from build123d import *

# Parameters (mm, degrees)
PAD_DEPTH           = 5
PAD001_DEPTH        = 10
POCKET_DEPTH        = 6
SKETCH003_W         = 7
SKETCH003_H         = 4
POCKET001_DEPTH     = 30
SKETCH004_W         = 15
SKETCH004_H         = 5
PAD002_DEPTH        = 10
SKETCH005_W         = 15
SKETCH005_H         = 55
PAD003_DEPTH        = 10
HOLE_D              = 3.4
HOLE_DEPTH          = 25
HOLE_CBORE_D        = 6.1
HOLE_CBORE_DEPTH    = 2.4
HOLE_TIPS_R         = 1.7
SKETCH007_W         = 15
SKETCH007_H         = 5
PAD004_DEPTH        = 10
SKETCH008_W         = 15
SKETCH008_H         = 55
PAD005_DEPTH        = 10
HOLE001_D           = 3.4
HOLE001_DEPTH       = 25
HOLE001_CBORE_D     = 6.1
HOLE001_CBORE_DEPTH = 2.4
HOLE001_TIPS_R      = 1.7
SKETCH010_W         = 15
SKETCH010_H         = 5
PAD006_DEPTH        = 10
SKETCH011_W         = 15
SKETCH011_H         = 55
PAD007_DEPTH        = 10
HOLE002_D           = 3.4
HOLE002_DEPTH       = 25
HOLE002_CBORE_D     = 6.1
HOLE002_CBORE_DEPTH = 2.4
HOLE002_TIPS_R      = 1.7


with BuildPart() as part:
    # Sketch → Pad (new body)
    with BuildSketch(Plane.XY):
        Polygon((77.465972, -44.725), (77.465972, -9.995), (87.465972, -9.995), (87.465972, -50.494492), (0, -100.995), (-87.465972, -50.494492), (-87.465972, 50.494492), (0, 100.995), (96.115509, 100.995), (89.45, 89.45), (0, 89.45), (-77.465972, 44.725), (-77.465972, -44.725), (0, -89.45), align=None)
    extrude(amount=PAD_DEPTH)

    # Sketch001 (on Face16 of Pad) → Pad001 (join)
    with BuildSketch(Plane.XY.offset(5)):
        Polygon((124.090672, 69.449404), (130.75638, 80.99429), (61.475035, 120.995481), (54.809328, 109.450596), align=None)
    extrude(amount=PAD001_DEPTH)

    # Sketch002 (on Face7 of Pad001) → Pocket (cut)
    with BuildSketch(Plane(origin=(0, 0, 5), x_dir=(1, 0, 0), z_dir=(0, 0, -1))):
        Polygon((91.032754, -92.191411), (117.013517, -77.191411), (120.513517, -83.253589), (94.532754, -98.253589), align=None)
    extrude(amount=-POCKET_DEPTH, mode=Mode.SUBTRACT)

    # Sketch003 (on Face8 of Pocket) → Pocket001 (cut)
    with BuildSketch(Plane(origin=(28.354514, -16.370486, 0), x_dir=(0.5, 0.866025, 0), z_dir=(0.866025, -0.5, 0))):
        with Locations((128.856481, 9)):
            Rectangle(SKETCH003_W, SKETCH003_H)
    extrude(amount=-POCKET001_DEPTH, mode=Mode.SUBTRACT)

    # Sketch004 (on Face14 of Pocket001) → Pad002 (join)
    with BuildSketch(Plane.YZ.offset(87.465972)):
        with Locations((-30.244746, 2.5)):
            Rectangle(SKETCH004_W, SKETCH004_H)
    extrude(amount=PAD002_DEPTH)

    # Sketch005 (on Face32 of Pad002) → Pad003 (join)
    with BuildSketch(Plane.YZ.offset(97.465972)):
        with Locations((-30.244746, -22.5)):
            Rectangle(SKETCH005_W, SKETCH005_H)
    extrude(amount=PAD003_DEPTH)

    # Hole
    with Locations(Plane.YZ.offset(107.465972)):
        with Locations((-30.244746, -12.5), (-30.244746, -37.5)):
            CounterBoreHole(HOLE_D / 2, HOLE_CBORE_D / 2, HOLE_CBORE_DEPTH, depth=HOLE_DEPTH)

    # Hole tips → Hole tip 1 section 0
    with BuildSketch(Plane.YZ.offset(82.465972), mode=Mode.PRIVATE) as hole_tip_1_s0:
        with Locations((-30.244746, -12.5)):
            Circle(HOLE_TIPS_R)
    loft([hole_tip_1_s0.sketch, Vertex(81.444509, -30.244746, -12.5)], mode=Mode.SUBTRACT)

    # Hole tips → Hole tip 2 section 0
    with BuildSketch(Plane.YZ.offset(82.465972), mode=Mode.PRIVATE) as hole_tip_2_s0:
        with Locations((-30.244746, -37.5)):
            Circle(HOLE_TIPS_R)
    loft([hole_tip_2_s0.sketch, Vertex(81.444509, -30.244746, -37.5)], mode=Mode.SUBTRACT)

    # Sketch007 (on Face17 of Hole) → Pad004 (join)
    with BuildSketch(Plane(origin=(43.732986, -75.744746, 0), x_dir=(0.866017, 0.500015, 0), z_dir=(0.500015, -0.866017, 0))):
        with Locations((0, 2.5)):
            Rectangle(SKETCH007_W, SKETCH007_H)
    extrude(amount=PAD004_DEPTH)

    # Sketch008 (on Face38 of Pad004) → Pad005 (join)
    with BuildSketch(Plane(origin=(48.733135, -84.404914, 0), x_dir=(0.866017, 0.500015, 0), z_dir=(0.500015, -0.866017, 0))):
        with Locations((0, -22.5)):
            Rectangle(SKETCH008_W, SKETCH008_H)
    extrude(amount=PAD005_DEPTH)

    # Hole001
    with Locations(Plane(origin=(53.733284, -93.065082, 0), x_dir=(0.866017, 0.500015, 0), z_dir=(0.500015, -0.866017, 0))):
        with Locations((0, -12.5), (0, -37.5)):
            CounterBoreHole(HOLE001_D / 2, HOLE001_CBORE_D / 2, HOLE001_CBORE_DEPTH, depth=HOLE001_DEPTH)

    # Hole001 tips → Hole001 tip 1 section 0
    with BuildSketch(Plane(origin=(41.232912, -71.414662, 0), x_dir=(0.866017, 0.500015, 0), z_dir=(0.500015, -0.866017, 0)), mode=Mode.PRIVATE) as hole001_tip_1_s0:
        with Locations((0, -12.5)):
            Circle(HOLE001_TIPS_R)
    loft([hole001_tip_1_s0.sketch, Vertex(40.722165, -70.530058, -12.5)], mode=Mode.SUBTRACT)

    # Hole001 tips → Hole001 tip 2 section 0
    with BuildSketch(Plane(origin=(41.232912, -71.414662, 0), x_dir=(0.866017, 0.500015, 0), z_dir=(0.500015, -0.866017, 0)), mode=Mode.PRIVATE) as hole001_tip_2_s0:
        with Locations((0, -37.5)):
            Circle(HOLE001_TIPS_R)
    loft([hole001_tip_2_s0.sketch, Vertex(40.722165, -70.530058, -37.5)], mode=Mode.SUBTRACT)

    # Sketch010 (on Face20 of Hole001) → Pad006 (join)
    with BuildSketch(Plane(origin=(-43.732986, -75.744746, 0), x_dir=(0.866017, -0.500015, 0), z_dir=(-0.500015, -0.866017, 0))):
        with Locations((0, 2.5)):
            Rectangle(SKETCH010_W, SKETCH010_H)
    extrude(amount=PAD006_DEPTH)

    # Sketch011 (on Face44 of Pad006) → Pad007 (join)
    with BuildSketch(Plane(origin=(-48.733135, -84.404914, 0), x_dir=(0.866017, -0.500015, 0), z_dir=(-0.500015, -0.866017, 0))):
        with Locations((0, -22.5)):
            Rectangle(SKETCH011_W, SKETCH011_H)
    extrude(amount=PAD007_DEPTH)

    # Hole002
    with Locations(Plane(origin=(-53.733284, -93.065082, 0), x_dir=(0.866017, -0.500015, 0), z_dir=(-0.500015, -0.866017, 0))):
        with Locations((0, -36.25), (0, -8.75)):
            CounterBoreHole(HOLE002_D / 2, HOLE002_CBORE_D / 2, HOLE002_CBORE_DEPTH, depth=HOLE002_DEPTH)

    # Hole002 tips → Hole002 tip 1 section 0
    with BuildSketch(Plane(origin=(-41.232912, -71.414662, 0), x_dir=(0.866017, -0.500015, 0), z_dir=(-0.500015, -0.866017, 0)), mode=Mode.PRIVATE) as hole002_tip_1_s0:
        with Locations((0, -36.25)):
            Circle(HOLE002_TIPS_R)
    loft([hole002_tip_1_s0.sketch, Vertex(-40.722165, -70.530058, -36.25)], mode=Mode.SUBTRACT)

    # Hole002 tips → Hole002 tip 2 section 0
    with BuildSketch(Plane(origin=(-41.232912, -71.414662, 0), x_dir=(0.866017, -0.500015, 0), z_dir=(-0.500015, -0.866017, 0)), mode=Mode.PRIVATE) as hole002_tip_2_s0:
        with Locations((0, -8.75)):
            Circle(HOLE002_TIPS_R)
    loft([hole002_tip_2_s0.sketch, Vertex(-40.722165, -70.530058, -8.75)], mode=Mode.SUBTRACT)


solid = part.part
The model under review builds one solid part; all positions refer to its coordinate system, in mm. A direction names the side the tool comes from. Give positions to 0.01 mm unless a question says otherwise; leave off trailing zeros. Loops run counter-clockwise (first coordinate to the right, second up) from the corner with the lowest first, then second, coordinate; pieces in that order, holes last. Notation, with made-up numbers: (51, 58.25) -> (80, 58.25) arc R18 ccw to (80, 83.25) -> close; hole circle Ø6 at (-31, -39.5). An arc over 180 degrees is marked (long way). Answer as a JSON object with one key per item and string values. Group by question number.
Q1. Take a section at C-C (y = 10). Write out the cut boundary in (x, z), plus the area to 3 significant figures.
Q2. Tool access review of faces 1 (the flat face through (-77.466, 1, 2)), 2 (the cylindrical face through (106.283, -27.336, -11.584)), 3 (the flat face through (80, 103, 7)): name each direction out of +Z, -Z, +X, -X, +Y, -Y from which nothing blocks a thin tool from reaching the whole face with its end or side.
Q3. Take a section at B-B (x = -30.5). Write out the cut boundary in (y, z), plus the area to 3 significant figures.
Q4. Insertion check: pin 1 (8 mm diameter, centred on x = 69, z = 6, fed in from -Y); pin 2 (1 mm diameter, centred on x = -57.5, z = -29.5, fed in from +Y); pin 3 (10 mm diameter, centred on x = 70.5, y = 114, fed in from -Z). Each pin has a flat end and moves straight along its axis. Give the tip position at first contact, or say it passes through.
Q5. Take a section at A-A (z = -23.5). Write out the cut boundary in (x, y).
Q6. Wall thickness on line 1 along X through (y, z) = (-89, -9); line 2 along Z through (x, y) = (7, 89.5); line 3 along Z through (x, y) = (102, 88): over which ranges is each line inside the solid? List them lowest first.
Q7. Draft analysis for pull direction Z (two halves, no side actions). For faces 4 (the flat face through (-48.824, -84.352, -24.65)), 5 (the flat face through (40, -67, 0)), 6 (the cylindrical face through (51.775, -86.975, -38.534)), state which applies: pulls with the +Z half, pulls with the -Z half, needs draft (parallel to the pull), parting line crosses it, or undercut.
Answer below:
{
 "1": {"outline": "(-87.47, 0) -> (-77.47, 0) -> (-77.47, 5) -> (-87.47, 5) -> close", "area": "50.0 mm2"},
 "2": {"face 1": "+Z, -Z", "face 2": "+X", "face 3": "none"},
 "3": {"outline": "(-83.39, 0) -> (-71.84, 0) -> (-71.84, 5) -> (-83.39, 5) -> close; (71.84, 0) -> (83.39, 0) -> (83.39, 5) -> (71.84, 5) -> close", "area": "115 mm2"},
 "4": {"pin 1": "stops at y = -63.39", "pin 2": "stops at y = -83.72", "pin 3": "stops at z = 5"},
 "5": {"outline": "(-60.23, -89.31) -> (-47.24, -96.82) -> (-42.24, -88.16) -> (-55.23, -80.65) -> close; (42.24, -88.16) -> (47.24, -96.82) -> (60.23, -89.31) -> (55.23, -80.65) -> close; (97.47, -37.74) -> (107.47, -37.74) -> (107.47, -22.74) -> (97.47, -22.74) -> close"},
 "6": {"line 1": "x = -60.05 to -53.33, -49.44 to -42.73, 42.73 to 60.05", "line 2": "z = 0 to 5", "line 3": "z = 11 to 15"},
 "7": {"face 4": "needs draft", "face 5": "pulls with the -Z half", "face 6": "undercut"}
}
